Here's how the part is built. I have some questions about the finished solid (model axes, mm). A direction names the side the tool comes from. Coordinates: 2 decimals unless noted, no trailing zeros. Write each loop counter-clockwise with the first axis right and the second up, starting at its lowest first coordinate (ties: lowest second). Pieces come first, ordered by that corner, then holes. Notation, with made-up numbers: (-30.75, 18) -> (3.25, 18) arc R21 cw to (3.25, 29) -> close; hole circle Ø11 at (46.5, -31.5). An arc over 180 degrees is marked (long way). Put each result on its own line as item: value. Start each with the question number.
Item 1: I want a section at A-A, the plane x = 18.5. List the corners of the cut face in (y, z) for me, then the cut area to 3 significant figures.
Item 2: On a 3-axis mill with a long thin cutter (end or side, diameter ignored), from which of +Z, -Z, +X, -X, +Y, -Y can I reach the whole of each face in a straight line? I mean faces 1 (the face through (4.93, 2.24, -13.3)), 2 (the face through (26.388, -39.384, -13.249)), 3 (the face through (15.21, 48.39, -12.59)). Say none if no direction works.
Item 3: If we mould it in two halves opening along Z, with no side actions, what happens to faces 4 (the face through (15.214, -33.481, 21.572)), 5 (the face through (30.86, 30, 19)), 6 (the face through (15.214, 46.548, 18.256)), 7 (the face through (15.21, -26.93, -42.13))? For each: released by +Z, released by -Z, zero draft, split by the parting line, or undercut.
Item 4: I want a section at C-C, the plane x = 8. List the corners of the cut face in (y, z) for me, then the cut area to 3 significant figures.
Item 5: I need wall thicknesses on line 1 (Y direction, x = 3, z = 8.5); line 2 (Z direction, x = 22, y = 7.5); line 3 (X direction, y = -16, z = -15). Which ranges of each line are inside material? Lowest first, please. Write a range as [from, to].
Item 6: I want a section at B-B, the plane x = 27.5. List the corners of the cut face in (y, z) for me.
Item 7: For pin 1 (6.5 mm diameter, centred on y = -7, z = -6.5, fed in from -X); pin 2 (6 mm diameter, centred on x = 22, z = 16.5, fed in from +Y); pin 3 (9 mm diameter, centred on y = -7.03, z = -6.44, fed in from +X), each with a flat end and sliding along its axis, tell me the tip position at first contact or that it passes through.
from build123d import *

# Parameters (mm, degrees)
SKETCH1_R           = 50
BOSS_EXTRUDE1_DEPTH = 30.86
SKETCH2_R           = 35
CUT_EXTRUDE1_DEPTH  = 8
CUT_EXTRUDE4_START  = -20
SKETCH10_W          = 10.01875972
SKETCH10_H          = 8.661840267
CUT_EXTRUDE4_DEPTH  = 60
SKETCH12_R          = 3.2
CUT_EXTRUDE5_DEPTH  = 2
SKETCH5_R           = 1.75
CUT_EXTRUDE3_DEPTH  = 30
SKETCH8_R           = 4
CUT_EXTRUDE6_DEPTH  = 10
SKETCH13_R          = 10
CUT_EXTRUDE8_DEPTH  = 40


with BuildPart() as part:
    # Sketch1 → Boss-Extrude1 (new body)
    with BuildSketch(Plane(origin=(0, 0, 0), x_dir=(0, 0, -1), z_dir=(1, 0, 0))):
        Circle(SKETCH1_R)
    extrude(amount=BOSS_EXTRUDE1_DEPTH)

    # Sketch2 → Cut-Extrude1 (cut)
    with BuildSketch(Plane(origin=(30.86, 0, 0), x_dir=(0, 0, -1), z_dir=(1, 0, 0))):
        Circle(SKETCH2_R)
    extrude(amount=-CUT_EXTRUDE1_DEPTH, mode=Mode.SUBTRACT)

    # Sketch10 → Cut-Extrude4 (cut)
    with BuildSketch(Plane(origin=(0, 0, 0), x_dir=(1, 0, 0), z_dir=(0, 0.976356599, 0.21616612)).offset(CUT_EXTRUDE4_START)):
        with Locations((27.048757514, 0.091052199)):
            Rectangle(SKETCH10_W, SKETCH10_H)
    extrude(amount=-CUT_EXTRUDE4_DEPTH, mode=Mode.SUBTRACT)

    # Sketch12 → Cut-Extrude5 (cut)
    with BuildSketch(Plane(origin=(22.86, 0, 0), x_dir=(0, 0, -1), z_dir=(1, 0, 0))):
        Circle(SKETCH12_R)
    extrude(amount=-CUT_EXTRUDE5_DEPTH, mode=Mode.SUBTRACT)

    # Sketch5 → Cut-Extrude3 (cut)
    with BuildSketch(Plane.ZY):
        with Locations((2.868272201, -9.088119419)):
            Circle(SKETCH5_R)
        with Locations((-6.436406189, -7.028056301)):
            Circle(SKETCH5_R)
        with Locations((-9.30467839, 2.060063119)):
            Circle(SKETCH5_R)
        with Locations((-2.868272201, 9.088119419)):
            Circle(SKETCH5_R)
        with Locations((6.436406189, 7.028056301)):
            Circle(SKETCH5_R)
        with Locations((9.30467839, -2.060063119)):
            Circle(SKETCH5_R)
    extrude(amount=-CUT_EXTRUDE3_DEPTH, mode=Mode.SUBTRACT)

    # Sketch8 → Cut-Extrude6 (cut)
    with BuildSketch(Plane.ZY):
        with Locations((-2.868272201, 9.088119419)):
            Circle(SKETCH8_R)
        with Locations((6.436406189, 7.028056301)):
            Circle(SKETCH8_R)
        with Locations((9.30467839, -2.060063119)):
            Circle(SKETCH8_R)
        with Locations((2.868272201, -9.088119419)):
            Circle(SKETCH8_R)
        with Locations((-6.436406189, -7.028056301)):
            Circle(SKETCH8_R)
        with Locations((-9.30467839, 2.060063119)):
            Circle(SKETCH8_R)
    extrude(amount=-CUT_EXTRUDE6_DEPTH, mode=Mode.SUBTRACT)

    # Sketch13 → Cut-Extrude8 (cut)
    with BuildSketch(Plane.ZY):
        with Locations((48.2405892, 12.470792391)):
            Circle(SKETCH13_R)
        with Locations((46.357604333, -18.266023916)):
            Circle(SKETCH13_R)
        with Locations((26.767590248, -42.025839926)):
            Circle(SKETCH13_R)
        with Locations((-3.046733515, -49.733213491)):
            Circle(SKETCH13_R)
        with Locations((-31.69730863, -38.444189871)):
            Circle(SKETCH13_R)
        with Locations((-48.2405892, -12.470792391)):
            Circle(SKETCH13_R)
        with Locations((-46.357604333, 18.266023916)):
            Circle(SKETCH13_R)
        with Locations((-26.767590248, 42.025839926)):
            Circle(SKETCH13_R)
        with Locations((3.046733515, 49.733213491)):
            Circle(SKETCH13_R)
        with Locations((31.69730863, 38.444189871)):
            Circle(SKETCH13_R)
    extrude(amount=-CUT_EXTRUDE8_DEPTH, mode=Mode.SUBTRACT)


solid = part.part
Calculated:
1. outline: (-49.51, 6.95) arc R10 cw to (-48.3, -12.94) arc R50 ccw to (-44.14, -23.48) arc R10 cw to (-31.46, -38.86) arc R50 ccw to (-21.91, -44.94) arc R10 cw to (-2.61, -49.93) arc R50 ccw to (8.69, -49.24) arc R10 cw to (27.23, -41.93) arc R50 ccw to (35.97, -34.73) arc R10 cw to (46.68, -17.92) arc R50 ccw to (49.51, -6.95) arc R10 cw to (48.3, 12.94) arc R50 ccw to (44.14, 23.48) arc R10 cw to (31.46, 38.86) arc R50 ccw to (21.91, 44.94) arc R10 cw to (2.61, 49.93) arc R50 ccw to (-8.69, 49.24) arc R10 cw to (-27.23, 41.93) arc R50 ccw to (-35.97, 34.73) arc R10 cw to (-46.68, 17.92) arc R50 ccw to start; hole circle Ø3.5 at (-9.09, 2.87); hole circle Ø3.5 at (-7.03, -6.44); hole circle Ø3.5 at (-2.06, 9.3); hole circle Ø3.5 at (2.06, -9.3); hole circle Ø3.5 at (7.03, 6.44); hole circle Ø3.5 at (9.09, -2.87)
1. area: 6,260 mm2
2. face 1: -X
2. face 2: +X, -Y
2. face 3: -Z, +X, -X, +Y
3. face 4: undercut
3. face 5: zero draft
3. face 6: released by +Z
3. face 7: released by -Z
4. outline: (-49.51, 6.95) arc R10 cw to (-48.3, -12.94) arc R50 ccw to (-44.14, -23.48) arc R10 cw to (-31.46, -38.86) arc R50 ccw to (-21.91, -44.94) arc R10 cw to (-2.61, -49.93) arc R50 ccw to (8.69, -49.24) arc R10 cw to (27.23, -41.93) arc R50 ccw to (35.97, -34.73) arc R10 cw to (46.68, -17.92) arc R50 ccw to (49.51, -6.95) arc R10 cw to (48.3, 12.94) arc R50 ccw to (44.14, 23.48) arc R10 cw to (31.46, 38.86) arc R50 ccw to (21.91, 44.94) arc R10 cw to (2.61, 49.93) arc R50 ccw to (-8.69, 49.24) arc R10 cw to (-27.23, 41.93) arc R50 ccw to (-35.97, 34.73) arc R10 cw to (-46.68, 17.92) arc R50 ccw to start; hole circle Ø8 at (-9.09, 2.87); hole circle Ø8 at (-7.03, -6.44); hole circle Ø8 at (-2.06, 9.3); hole circle Ø8 at (2.06, -9.3); hole circle Ø8 at (7.03, 6.44); hole circle Ø8 at (9.09, -2.87)
4. area: 6,010 mm2
5. line 1: y = [-49.27, -5.98], [1.86, 3.6], [10.45, 41.35]
5. line 2: z = [-49.43, -3.6], [-2.13, 4.75], [8.12, 39.56]
5. line 3: x = [0, 22.86]
6. outline: (-49.51, 6.95) arc R10 cw to (-39.84, -4.48) -> (-34.84, -3.37) arc R35 cw (long way) to (-32.94, -11.82) -> (-47.67, -15.08) arc R50 ccw to (-44.14, -23.48) arc R10 cw to (-31.46, -38.86) arc R50 ccw to (-21.91, -44.94) arc R10 cw to (-2.61, -49.93) arc R50 ccw to (8.69, -49.24) arc R10 cw to (27.23, -41.93) arc R50 ccw to (35.97, -34.73) arc R10 cw to (46.68, -17.92) arc R50 ccw to (49.51, -6.95) arc R10 cw to (48.3, 12.94) arc R50 ccw to (44.14, 23.48) arc R10 cw to (31.46, 38.86) arc R50 ccw to (21.91, 44.94) arc R10 cw to (2.61, 49.93) arc R50 ccw to (-8.69, 49.24) arc R10 cw to (-27.23, 41.93) arc R50 ccw to (-35.97, 34.73) arc R10 cw to (-46.68, 17.92) arc R50 ccw to start
7. pin 1: stops at x = 10
7. pin 2: stops at y = 48.14
7. pin 3: stops at x = 22.86
